Geometry check sheet. Reference: drawing and pictorial views, mm from the part's lowest x, y, z. Coordinates: 2 decimals unless noted, no trailing zeros. Write each loop counter-clockwise with the first axis right and the second up, starting at its lowest first coordinate (ties: lowest second). Pieces come first, ordered by that corner, then holes. Notation, with made-up numbers: (14.5, 30) - (66.5, 30) arc R23 cw to (66.5, 49) - close; hole circle Ø6 at (-12.5, 87). An arc over 180 degrees is marked (long way). Answer as a JSON object with one key per item and string values. Group by question number.
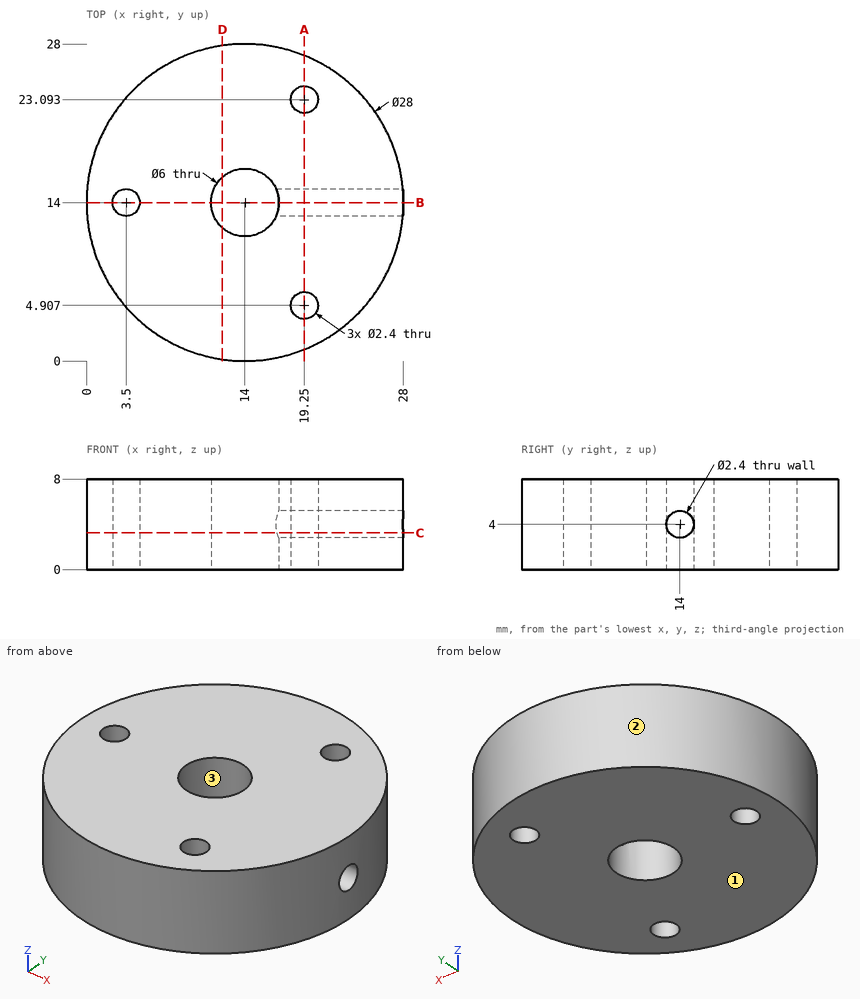
(1) Section check D-D (x = 12). Record the cut outline in (y, z), and give its area (3 significant figures).
(2) Draft check along Y on the marked faces 1, 2 and 3. Enter one of: +Y half, -Y half, draft (parallel to the pull), parting line (faces both ways), or undercut.
(3) Gauge pin test, flat ends, axial feed: pin 1 (3 mm diameter, centred on y = 8.5, z = 3.5, fed in from -X); pin 2 (3 mm diameter, centred on x = 19.25, y = 23.09, fed in from +Z); pin 3 (1.9 mm diameter, centred on y = 14, z = 4, fed in from +X); pin 4 (1.9 mm diameter, centred on x = 3.5, y = 14, fed in from +Z). Record the tip position at first contact, or that the pin passes through.
(4) Section check C-C (z = 3.25). Record the cut outline in (x, y), and give its area (3 significant figures).
(5) Section check B-B (y = 14). Record the cut outline in (x, z).
(6) Material ranges on L1, parallel to Y at x = 14, z = 1.75; L2, parallel to Y at x = 19.25, z = 5 (1 decimal); L3, parallel to Y at x = 12, z = 7.5 (1 decimal), recorded low to high. Write a range as [from, to].
(7) Section check A-A (x = 19.25). Record the cut outline in (y, z).
Conclusion:
{
 "1": {"outline": "(0.14, 0) - (11.76, 0) - (11.76, 8) - (0.14, 8) - close; (16.24, 0) - (27.86, 0) - (27.86, 8) - (16.24, 8) - close", "area": "186 mm^2"},
 "2": {"face 1": "draft", "face 2": "parting line", "face 3": "undercut"},
 "3": {"pin 1": "stops at x = 0.58", "pin 2": "stops at z = 8", "pin 3": "stops at x = 11.15", "pin 4": "passes through"},
 "4": {"outline": "(16.85, 13.06) arc R3 cw (long way) to (16.85, 14.94) - (27.97, 14.94) arc R14 ccw (long way) to (27.97, 13.06) - close; hole circle Ø2.4 at (3.5, 14); hole circle Ø2.4 at (19.25, 4.91); hole circle Ø2.4 at (19.25, 23.09)", "area": "553 mm^2"},
 "5": {"outline": "(0, 0) - (2.3, 0) - (2.3, 8) - (0, 8) - close; (4.7, 0) - (11, 0) - (11, 8) - (4.7, 8) - close; (17, 0) - (28, 0) - (28, 2.8) - (17, 2.8) - close; (17, 5.2) - (28, 5.2) - (28, 8) - (17, 8) - close"},
 "6": {"L1": "y = [0, 11], [17, 28]", "L2": "y = [1, 3.7], [6.1, 13.3], [14.7, 21.9], [24.3, 27]", "L3": "y = [0.1, 11.8], [16.2, 27.9]"},
 "7": {"outline": "(1.02, 0) - (3.71, 0) - (3.71, 8) - (1.02, 8) - close; (6.11, 0) - (21.89, 0) - (21.89, 8) - (6.11, 8) - close; (24.29, 0) - (26.98, 0) - (26.98, 8) - (24.29, 8) - close; hole circle Ø2.4 at (14, 4)"}
}
